```python
from build123d import *

# Parameters (mm, degrees)
CYLINDER002_R     = 1.65
CYLINDER002_DEPTH = 10
BOX005_W          = 7
BOX005_H          = 5
BOX005_DEPTH      = 12
BOX006_W          = 14
BOX006_H          = 3
BOX006_DEPTH      = 12
BOX007_W          = 2
BOX007_H          = 5
BOX007_DEPTH      = 12
BOX008_W          = 14
BOX008_H          = 3
BOX008_DEPTH      = 12
BOX009_W          = 2
BOX009_H          = 5
BOX009_DEPTH      = 12
BOX010_W          = 7
BOX010_H          = 2
BOX010_DEPTH      = 7.8
CHAMFER006_SIZE   = 1
CHAMFER007_SIZE   = 0.4
CHAMFER008_SIZE   = 0.4


with BuildPart() as cylinder002:
    # Cylinder002 → Cylinder002 (new body)
    with BuildSketch(Plane(origin=(0, 0, 6), x_dir=(1, 0, 0), z_dir=(0, 1, 0))):
        Circle(CYLINDER002_R)
    extrude(amount=CYLINDER002_DEPTH)


with BuildPart() as cube005:
    # Box005 → Box005 (new body)
    with BuildSketch(Plane(origin=(-3.5, 0, 0), x_dir=(1, 0, 0), z_dir=(0, 0, 1))):
        with Locations((3.5, 2.5)):
            Rectangle(BOX005_W, BOX005_H)
    extrude(amount=BOX005_DEPTH)


with BuildPart() as cube006:
    # Box006 → Box006 (new body)
    with BuildSketch(Plane(origin=(3.5, 0, 0), x_dir=(1, 0, 0), z_dir=(0, 0, 1))):
        with Locations((7, 1.5)):
            Rectangle(BOX006_W, BOX006_H)
    extrude(amount=BOX006_DEPTH)


with BuildPart() as cube007:
    # Box007 → Box007 (new body)
    with BuildSketch(Plane(origin=(17.5, 0, 0), x_dir=(1, 0, 0), z_dir=(0, 0, 1))):
        with Locations((1, 2.5)):
            Rectangle(BOX007_W, BOX007_H)
    extrude(amount=BOX007_DEPTH)


with BuildPart() as cube008:
    # Box008 → Box008 (new body)
    with BuildSketch(Plane(origin=(-17.5, 0, 0), x_dir=(1, 0, 0), z_dir=(0, 0, 1))):
        with Locations((7, 1.5)):
            Rectangle(BOX008_W, BOX008_H)
    extrude(amount=BOX008_DEPTH)


with BuildPart() as cube009:
    # Box009 → Box009 (new body)
    with BuildSketch(Plane(origin=(-19.5, 0, 0), x_dir=(1, 0, 0), z_dir=(0, 0, 1))):
        with Locations((1, 2.5)):
            Rectangle(BOX009_W, BOX009_H)
    extrude(amount=BOX009_DEPTH)


with BuildPart() as chamfer008:
    # Box010 → Box010 (new body)
    with BuildSketch(Plane(origin=(-3.5, 4, 2.1), x_dir=(1, 0, 0), z_dir=(0, 0, 1))):
        with Locations((3.5, 1)):
            Rectangle(BOX010_W, BOX010_H)
    extrude(amount=BOX010_DEPTH)

    # Fusion003: union Cube005, Cube006, Cube007, Cube008, Cube009
    add(cube005.part)
    add(cube006.part)
    add(cube007.part)
    add(cube008.part)
    add(cube009.part)

    # Cut003: cut Cylinder002
    add(cylinder002.part, mode=Mode.SUBTRACT)

    # Chamfer006
    chamfer006_edges = [chamfer008.edges().sort_by_distance(p)[0] for p in [
        (-19.5, 0, 6),
        (19.5, 0, 6),
    ]]
    chamfer(chamfer006_edges, length=CHAMFER006_SIZE)

    # Chamfer007
    chamfer007_edges = [chamfer008.edges().sort_by_distance(p)[0] for p in [
        (-19.5, 5, 6),
        (-17.5, 5, 6),
        (19.5, 5, 6),
        (17.5, 5, 6),
    ]]
    chamfer(chamfer007_edges, length=CHAMFER007_SIZE)

    # Chamfer008
    chamfer008_edges = [chamfer008.edges().sort_by_distance(p)[0] for p in [
        (-19.5, 2.8, 12),
        (-19.5, 2.8, 0),
        (-19, 0.5, 12),
        (0, 0, 12),
        (19, 0.5, 12),
        (19.5, 2.8, 12),
        (19.3, 4.8, 12),
        (18.5, 5, 12),
        (17.7, 4.8, 12),
        (17.5, 3.8, 12),
        (10.5, 3, 12),
        (3.5, 4, 12),
        (0, 5, 12),
        (-3.5, 4, 12),
        (-10.5, 3, 12),
        (-17.5, 3.8, 12),
        (-17.7, 4.8, 12),
        (-18.5, 5, 12),
        (-19.3, 4.8, 12),
        (-19.3, 4.8, 0),
        (-19, 0.5, 0),
        (19.5, 2.8, 0),
        (19, 0.5, 0),
        (0, 0, 0),
        (-18.5, 5, 0),
        (-17.7, 4.8, 0),
        (-17.5, 3.8, 0),
        (-10.5, 3, 0),
        (-3.5, 4, 0),
        (0, 5, 0),
        (3.5, 4, 0),
        (10.5, 3, 0),
        (17.5, 3.8, 0),
        (17.7, 4.8, 0),
        (18.5, 5, 0),
        (19.3, 4.8, 0),
    ]]
    chamfer(chamfer008_edges, length=CHAMFER008_SIZE)


solid = chamfer008.part
```
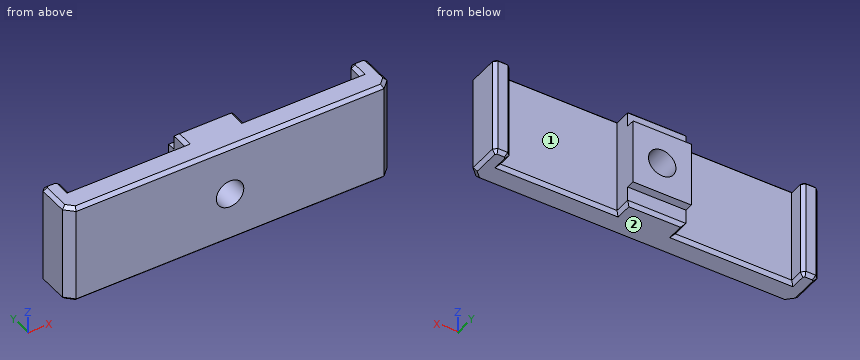
The model under review builds one solid part; all positions refer to its coordinate system, in mm. Face numbers are marked on the shaded views. A direction names the side the tool comes from. Give positions to 0.01 mm unless a question says otherwise; leave off trailing zeros. Write each loop counter-clockwise with the first axis right and the second up, starting at its lowest first coordinate (ties: lowest second). Pieces come first, ordered by that corner, then holes.
(1) To check wall thickness, follow L1, parallel to X at y = 3.25, z = 9; L2, parallel to X at y = 2, z = 6; L3, parallel to Z at x = 0, y = 2.2. State the ranges of each line that lie inside material, in increasing order.
(2) Consider section C-C, the plane y = 2.25. Give the boundary of the cut face in (x, z), and give its area (3 significant figures).
(3) Consider section B-B, the plane x = 0. Give the boundary of the cut face in (y, z).
(4) Consider section D-D, the plane x = -7.5. Give the boundary of the cut face in (y, z).
(5) For P1, Ø0.6, axis at x = -19, z = 7, coming from the +Y side; P2, Ø3.5, axis at x = -12, z = 8, coming from the +Y side; P3, Ø0.5, axis at x = -1, y = 5.5, coming from the +Z side, all flat-tipped, find the tip position at first contact; note any pin that passes through.
(6) Tool access review of the marked faces 1 and 2: name each direction out of +Z, -Z, +X, -X, +Y, -Y from which nothing blocks a thin tool from reaching the whole face with its end or side.
(7) Consider section A-A, the plane z = 6. Give the boundary of the cut face in (x, y).
Returned:
1. L1: x = -19.5 to -17.5, -3.5 to 3.5, 17.5 to 19.5
1. L2: x = -19.5 to -1.65, 1.65 to 19.5
1. L3: z = 0 to 4.35, 7.65 to 12
2. outline: (-19.5, 0.4) - (-19.1, 0) - (19.1, 0) - (19.5, 0.4) - (19.5, 11.6) - (19.1, 12) - (-19.1, 12) - (-19.5, 11.6) - close; hole circle Ø3.3 at (0, 6)
2. area: 459 mm2
3. outline: (0, 0.4) - (0.4, 0) - (4.6, 0) - (5, 0.4) - (5, 2.1) - (6, 2.1) - (6, 4.35) - (0, 4.35) - close; (0, 7.65) - (6, 7.65) - (6, 9.9) - (5, 9.9) - (5, 11.6) - (4.6, 12) - (0.4, 12) - (0, 11.6) - close
4. outline: (0, 0.4) - (0.4, 0) - (2.6, 0) - (3, 0.4) - (3, 11.6) - (2.6, 12) - (0.4, 12) - (0, 11.6) - close
5. P1: stops at y = 5
5. P2: stops at y = 3
5. P3: stops at z = 9.9
6. face 1: +Z, -Z, +Y
6. face 2: -Z, +X, -X, +Y, -Y
7. outline: (-19.5, 1) - (-18.5, 0) - (-1.65, 0) - (-1.65, 6) - (-3.5, 6) - (-3.5, 3) - (-17.5, 3) - (-17.5, 4.6) - (-17.9, 5) - (-19.1, 5) - (-19.5, 4.6) - close; (1.65, 0) - (18.5, 0) - (19.5, 1) - (19.5, 4.6) - (19.1, 5) - (17.9, 5) - (17.5, 4.6) - (17.5, 3) - (3.5, 3) - (3.5, 6) - (1.65, 6) - close
